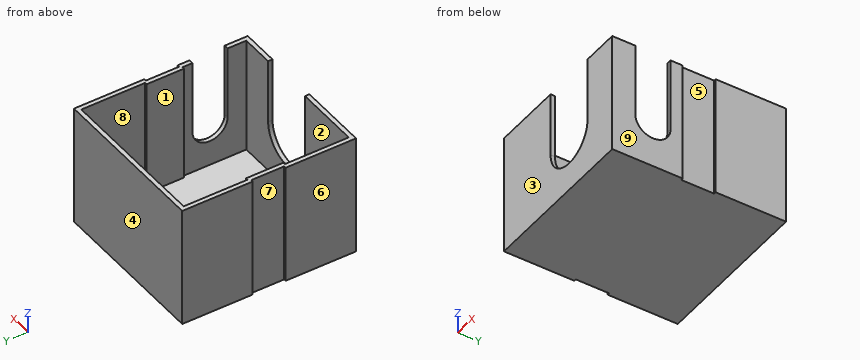
```python
from build123d import *

# Parameters (mm, degrees)
F1_DEPTH = 2
F2_DEPTH = 55
F4_DEPTH = 3
F6_DEPTH = 3


with BuildPart() as f1:
    # F0 (on Top) → F1 (new body)
    with BuildSketch(Plane.XY):
        Polygon((-35, -37.5), (35, -37.5), (35, -8.5), (34, -8.5), (34, 0), (34, 8.5), (35, 8.5), (35, 37.5), (-35, 37.5), (-35, 8.5), (-34, 8.5), (-34, 0), (-34, -8.5), (-35, -8.5), align=None)
    extrude(amount=F1_DEPTH)

    # F0 (on Top) → F2 (join)
    with BuildSketch(Plane.XY):
        Polygon((-37, -39.5), (37, -39.5), (37, -7.5), (36, -7.5), (36, 0), (36, 7.5), (37, 7.5), (37, 39.5), (-37, 39.5), (-37, 7.5), (-36, 7.5), (-36, 0), (-36, -7.5), (-37, -7.5), align=None)
        Polygon((35, -8.5), (35, -37.5), (-35, -37.5), (-35, -8.5), (-34, -8.5), (-34, 0), (-34, 8.5), (-35, 8.5), (-35, 37.5), (35, 37.5), (35, 8.5), (34, 8.5), (34, 0), (34, -8.5), align=None, mode=Mode.SUBTRACT)
    extrude(amount=F2_DEPTH)

    # F3 (on face) → F4 (cut)
    with BuildSketch(Plane.XZ.offset(39.5)):
        with BuildLine():
            Line((-5.120877, 55), (-5.120877, 25.502008))
            ThreePointArc((-5.120877, 25.502008), (7.485725, 12.895406), (20.092327, 25.502008))
            Line((20.092327, 25.502008), (20.092327, 55))
            Line((20.092327, 55), (-5.120877, 55))
        make_face()
    extrude(amount=-F4_DEPTH, mode=Mode.SUBTRACT)

    # F5 (on face) → F6 (cut)
    with BuildSketch(Plane.YZ.offset(37)):
        with BuildLine():
            ThreePointArc((-28.975196, 21.504425), (-20.975196, 13.504425), (-12.975196, 21.504425))
            Line((-12.975196, 21.504425), (-12.975196, 55))
            Line((-12.975196, 55), (-28.975196, 55))
            Line((-28.975196, 55), (-28.975196, 21.504425))
        make_face()
    extrude(amount=-F6_DEPTH, mode=Mode.SUBTRACT)


solid = f1.part
```
Could you check a few things on this model? Use its own coordinates, in mm. Face numbers are marked on the shaded views. A direction names the side the tool comes from. Round coordinates to 2 decimals unless told otherwise and drop trailing zeros. Write each loop counter-clockwise with the first axis right and the second up, starting at its lowest first coordinate (ties: lowest second). Pieces come first, ordered by that corner, then holes. Notation, with made-up numbers: M -38,16.5 L -24,16.5 A21 cw -24,28.5 Z; hole C -27,69.25 d6. An arc over 180 degrees is marked long. Write each question's results on one line, items separated by ' | '. Start each with the question number.
1. Thinking about a two-plate mould opening in Y: for the marked faces 1, 2, 3 and 4, which applies, +Y half, -Y half, draft (parallel to the pull), parting line (faces both ways), or undercut?
2. Imagine slicing it at C-C on x = -13. List the corners of the cut face in (y, z) for me, and give its area (3 significant figures).
3. Imagine slicing it at D-D on z = 11. List the corners of the cut face in (x, y) for me.
4. Imagine slicing it at B-B on y = 32.5. List the corners of the cut face in (x, z) for me, and give its area (3 significant figures).
5. On a 3-axis mill with a long thin cutter (end or side, diameter ignored), from which of +Z, -Z, +X, -X, +Y, -Y can I reach the whole of each face in a straight line? I mean the marked faces 5, 6, 7, 8 and 9. Say none if no direction works.
6. I need wall thicknesses on L1, parallel to Y at x = 24.5, z = 19; L2, parallel to X at y = 30, z = 33.5; L3, parallel to X at y = 5.5, z = 14. Which ranges of each line are inside material? Lowest first, please. Write a range as from..to.
7. I'm going to push a flat-ended pin straight in: pin 1 Ø7.5 at (y, z) = (-0.5, 24.5) entering from +X. Where does the tip first touch, or does it pass through?
Result sheet:
1) face 1: undercut | face 2: undercut | face 3: -Y half | face 4: +Y half
2) outline: M -39.5,0 L 39.5,0 L 39.5,55 L 37.5,55 L 37.5,2 L -37.5,2 L -37.5,55 L -39.5,55 Z | area: 370 mm^2
3) outline: M -37,-39.5 L 37,-39.5 L 37,-7.5 L 36,-7.5 L 36,7.5 L 37,7.5 L 37,39.5 L -37,39.5 L -37,7.5 L -36,7.5 L -36,-7.5 L -37,-7.5 Z; hole M -35,-37.5 L 35,-37.5 L 35,-8.5 L 34,-8.5 L 34,8.5 L 35,8.5 L 35,37.5 L -35,37.5 L -35,8.5 L -34,8.5 L -34,-8.5 L -35,-8.5 Z
4) outline: M -37,0 L 37,0 L 37,55 L 35,55 L 35,2 L -35,2 L -35,55 L -37,55 Z | area: 360 mm^2
5) face 5: +Z, -Z, +X | face 6: +Z, -Z, -X, +Y, -Y | face 7: +Z, -Z, -X | face 8: +Z | face 9: +Z, -Z, +X, +Y, -Y
6) L1: y = -39.5..-37.5, 37.5..39.5 | L2: x = -37..-35, 35..37 | L3: x = -36..-34, 34..36
7) pin 1: stops at x = 36
